from build123d import *

# Parameters (mm, degrees)
BOSS_EXTRUDE1_DEPTH            = 20
M3_CLEARANCE_HOLE1_D           = 3.2
M3_CLEARANCE_HOLE1_CSINK_D     = 3.45
M3_CLEARANCE_HOLE1_CSINK_ANGLE = 90


with BuildPart() as part:
    # Sketch1 → Boss-Extrude1 (new body)
    with BuildSketch(Plane.XY):
        Polygon((0, 44), (24, 44), (24, 0), (57, 0), (57, 3), (27, 3), (27, 47), (0, 47), align=None)
    extrude(amount=BOSS_EXTRUDE1_DEPTH)

    # M3 Clearance Hole1 (through all)
    with Locations(Plane(origin=(0, 47, 0), x_dir=(1, 0, 0), z_dir=(0, 1, 0))):
        with Locations((15, -15), (5, -5), (5, -15), (15, -5)):
            CounterSinkHole(M3_CLEARANCE_HOLE1_D / 2, M3_CLEARANCE_HOLE1_CSINK_D / 2, counter_sink_angle=M3_CLEARANCE_HOLE1_CSINK_ANGLE)


solid = part.part
Build history of the part. All positions in model axes, mm. A direction names the side the tool comes from. Round coordinates to 2 decimals unless told otherwise and drop trailing zeros. Write each loop counter-clockwise with the first axis right and the second up, starting at its lowest first coordinate (ties: lowest second). Pieces come first, ordered by that corner, then holes. Notation, with made-up numbers: (29.25, 43.25) - (88.25, 43.25) arc R23 cw to (88.25, 62.25) - close; hole circle Ø4 at (20.5, 64). An arc over 180 degrees is marked (long way). Use CSV: the item, a comma, the result in double quotes.
(1) Band-saw the part on A-A (z = 15). Write the cut outline in (x, y) (3 decimals).
Response:
outline,"(0, 44) - (3.4, 44) - (3.4, 46.875) - (3.275, 47) - (0, 47) - close; (6.6, 44) - (13.4, 44) - (13.4, 46.875) - (13.275, 47) - (6.725, 47) - (6.6, 46.875) - close; (16.6, 44) - (24, 44) - (24, 0) - (57, 0) - (57, 3) - (27, 3) - (27, 47) - (16.725, 47) - (16.6, 46.875) - close"
(2) Wall check: line 1 (X direction, y = 45.7, z = 15); line 2 (Z direction, x = 5, y = 46); line 3 (X direction, y = 4, z = 2.25). Give the ranges that are in metal, low to high.
Response:
line 1,"0 to 3.4, 6.6 to 13.4, 16.6 to 27"
line 2,"0 to 3.4, 6.6 to 13.4, 16.6 to 20"
line 3,"24 to 27"
(3) Band-saw the part on D-D (y = 31). Write the cut outline in (x, z), plus the area to 3 significant figures.
Response:
outline,"(24, 0) - (27, 0) - (27, 20) - (24, 20) - close"
area,"60.0 mm²"
(4) 3-axis set-ups, long thin cutter, end or side, ignore diameter. For faces 4 (the flat face through (24, 22, 10)), 5 (the flat face through (40, 0, 10)), 6 (the flat face through (27, 25, 10)): which of +Z, -Z, +X, -X, +Y, -Y reach the whole face in a straight line?
Response:
face 4,"+Z, -Z, -X, -Y"
face 5,"+Z, -Z, +X, -X, -Y"
face 6,"+Z, -Z, +X, +Y"
(5) Band-saw the part on B-B (x = 5). Write the cut outline in (y, z) (3 decimals).
Response:
outline,"(44, 0) - (47, 0) - (47, 3.275) - (46.875, 3.4) - (44, 3.4) - close; (44, 6.6) - (46.875, 6.6) - (47, 6.725) - (47, 13.275) - (46.875, 13.4) - (44, 13.4) - close; (44, 16.6) - (46.875, 16.6) - (47, 16.725) - (47, 20) - (44, 20) - close"
(6) Mould opens along Z. For faces 1 (the flat face through (12, 44, 10)), 2 (the flat face through (26, 24, 20)), 3 (the cylindrical face through (16.6, 45.42, 4.93)) say: pulls with the +Z half, pulls with the -Z half, needs draft (parallel to the pull), parting line crosses it, or undercut.
Response:
face 1,"needs draft"
face 2,"pulls with the +Z half"
face 3,"undercut"
(7) Pin check, flat tips, straight feed: P1, Ø5, axis at x = 44.5, z = 4.5, coming from the +Y side; P2, Ø3, axis at y = 22, z = 15, coming from the +X side; P3, Ø1.5, axis at y = 5.5, z = 4, coming from the -X side. Stop position of each tip, or through.
Response:
P1,"y = 3"
P2,"x = 27"
P3,"x = 24"
(8) Band-saw the part on C-C (z = 10.5). Write the cut outline in (x, y), plus the area to 3 significant figures.
Response:
outline,"(0, 44) - (24, 44) - (24, 0) - (57, 0) - (57, 3) - (27, 3) - (27, 47) - (0, 47) - close"
area,"303 mm²"
